```python
from build123d import *

# Parameters (mm, degrees)
SKETCH_1_W                        = 10
SKETCH_1_H                        = 10
EXTRUDE_1_DEPTH                   = 1
SKETCH_2_R                        = 0.5
EXTRUDE_2_DEPTH                   = 5
PATTERN_LINEAR_1_COUNT            = 5
PATTERN_LINEAR_1_PITCH            = 2
PATTERN_LINEAR_2_COUNT            = 5
PATTERN_LINEAR_2_PITCH            = 2
PATTERN_LINEAR_2_COPY_1_SKETCH_R  = 0.5
PATTERN_LINEAR_2_COPY_1_DEPTH     = 5
PATTERN_LINEAR_2_COPY_2_SKETCH_R  = 0.5
PATTERN_LINEAR_2_COPY_2_DEPTH     = 5
PATTERN_LINEAR_2_COPY_3_SKETCH_R  = 0.5
PATTERN_LINEAR_2_COPY_3_DEPTH     = 5
PATTERN_LINEAR_2_COPY_4_SKETCH_R  = 0.5
PATTERN_LINEAR_2_COPY_4_DEPTH     = 5
PATTERN_LINEAR_2_COPY_5_SKETCH_R  = 0.5
PATTERN_LINEAR_2_COPY_5_DEPTH     = 5
PATTERN_LINEAR_2_COPY_6_SKETCH_R  = 0.5
PATTERN_LINEAR_2_COPY_6_DEPTH     = 5
PATTERN_LINEAR_2_COPY_7_SKETCH_R  = 0.5
PATTERN_LINEAR_2_COPY_7_DEPTH     = 5
PATTERN_LINEAR_2_COPY_8_SKETCH_R  = 0.5
PATTERN_LINEAR_2_COPY_8_DEPTH     = 5
PATTERN_LINEAR_2_COPY_9_SKETCH_R  = 0.5
PATTERN_LINEAR_2_COPY_9_DEPTH     = 5
PATTERN_LINEAR_2_COPY_10_SKETCH_R = 0.5
PATTERN_LINEAR_2_COPY_10_DEPTH    = 5
PATTERN_LINEAR_2_COPY_11_SKETCH_R = 0.5
PATTERN_LINEAR_2_COPY_11_DEPTH    = 5
PATTERN_LINEAR_2_COPY_12_SKETCH_R = 0.5
PATTERN_LINEAR_2_COPY_12_DEPTH    = 5
PATTERN_LINEAR_2_COPY_13_SKETCH_R = 0.5
PATTERN_LINEAR_2_COPY_13_DEPTH    = 5
PATTERN_LINEAR_2_COPY_14_SKETCH_R = 0.5
PATTERN_LINEAR_2_COPY_14_DEPTH    = 5
PATTERN_LINEAR_2_COPY_15_SKETCH_R = 0.5
PATTERN_LINEAR_2_COPY_15_DEPTH    = 5
PATTERN_LINEAR_2_COPY_16_SKETCH_R = 0.5
PATTERN_LINEAR_2_COPY_16_DEPTH    = 5


with BuildPart() as part:
    # 草圖1 → 填料-伸長1 (new body)
    with BuildSketch(Plane(origin=(0, 0, 0), x_dir=(1, 0, 0), z_dir=(0, 1, 0))):
        Rectangle(SKETCH_1_W, SKETCH_1_H)
    extrude(amount=EXTRUDE_1_DEPTH)

    # 草圖2 → 填料-伸長2 (add)
    with BuildSketch(Plane(origin=(0, 1, 0), x_dir=(1, 0, 0), z_dir=(0, 1, 0))):
        with Locations(Location((-4, 4, 0), (0, 0, 90))):
            Circle(SKETCH_2_R)
    extrude_2 = extrude(amount=EXTRUDE_2_DEPTH)

    # 直線複製排列1: 填料-伸長2 ×5
    with Locations(*[(i * PATTERN_LINEAR_1_PITCH, 0, 0) for i in range(1, PATTERN_LINEAR_1_COUNT)]):
        add(extrude_2)

    # 直線複製排列2: 填料-伸長2 ×5
    with Locations(*[(0, 0, i * PATTERN_LINEAR_2_PITCH) for i in range(1, PATTERN_LINEAR_2_COUNT)]):
        add(extrude_2)

    # 直線複製排列2 copy 1 sketch → 直線複製排列2 copy 1 (add)
    with BuildSketch(Plane(origin=(2, 1, 2), x_dir=(1, 0, 0), z_dir=(0, 1, 0))):
        with Locations(Location((-4, 4, 0), (0, 0, 90))):
            Circle(PATTERN_LINEAR_2_COPY_1_SKETCH_R)
    extrude(amount=PATTERN_LINEAR_2_COPY_1_DEPTH)

    # 直線複製排列2 copy 2 sketch → 直線複製排列2 copy 2 (add)
    with BuildSketch(Plane(origin=(2, 1, 4), x_dir=(1, 0, 0), z_dir=(0, 1, 0))):
        with Locations(Location((-4, 4, 0), (0, 0, 90))):
            Circle(PATTERN_LINEAR_2_COPY_2_SKETCH_R)
    extrude(amount=PATTERN_LINEAR_2_COPY_2_DEPTH)

    # 直線複製排列2 copy 3 sketch → 直線複製排列2 copy 3 (add)
    with BuildSketch(Plane(origin=(2, 1, 6), x_dir=(1, 0, 0), z_dir=(0, 1, 0))):
        with Locations(Location((-4, 4, 0), (0, 0, 90))):
            Circle(PATTERN_LINEAR_2_COPY_3_SKETCH_R)
    extrude(amount=PATTERN_LINEAR_2_COPY_3_DEPTH)

    # 直線複製排列2 copy 4 sketch → 直線複製排列2 copy 4 (add)
    with BuildSketch(Plane(origin=(2, 1, 8), x_dir=(1, 0, 0), z_dir=(0, 1, 0))):
        with Locations(Location((-4, 4, 0), (0, 0, 90))):
            Circle(PATTERN_LINEAR_2_COPY_4_SKETCH_R)
    extrude(amount=PATTERN_LINEAR_2_COPY_4_DEPTH)

    # 直線複製排列2 copy 5 sketch → 直線複製排列2 copy 5 (add)
    with BuildSketch(Plane(origin=(4, 1, 2), x_dir=(1, 0, 0), z_dir=(0, 1, 0))):
        with Locations(Location((-4, 4, 0), (0, 0, 90))):
            Circle(PATTERN_LINEAR_2_COPY_5_SKETCH_R)
    extrude(amount=PATTERN_LINEAR_2_COPY_5_DEPTH)

    # 直線複製排列2 copy 6 sketch → 直線複製排列2 copy 6 (add)
    with BuildSketch(Plane(origin=(4, 1, 4), x_dir=(1, 0, 0), z_dir=(0, 1, 0))):
        with Locations(Location((-4, 4, 0), (0, 0, 90))):
            Circle(PATTERN_LINEAR_2_COPY_6_SKETCH_R)
    extrude(amount=PATTERN_LINEAR_2_COPY_6_DEPTH)

    # 直線複製排列2 copy 7 sketch → 直線複製排列2 copy 7 (add)
    with BuildSketch(Plane(origin=(4, 1, 6), x_dir=(1, 0, 0), z_dir=(0, 1, 0))):
        with Locations(Location((-4, 4, 0), (0, 0, 90))):
            Circle(PATTERN_LINEAR_2_COPY_7_SKETCH_R)
    extrude(amount=PATTERN_LINEAR_2_COPY_7_DEPTH)

    # 直線複製排列2 copy 8 sketch → 直線複製排列2 copy 8 (add)
    with BuildSketch(Plane(origin=(4, 1, 8), x_dir=(1, 0, 0), z_dir=(0, 1, 0))):
        with Locations(Location((-4, 4, 0), (0, 0, 90))):
            Circle(PATTERN_LINEAR_2_COPY_8_SKETCH_R)
    extrude(amount=PATTERN_LINEAR_2_COPY_8_DEPTH)

    # 直線複製排列2 copy 9 sketch → 直線複製排列2 copy 9 (add)
    with BuildSketch(Plane(origin=(6, 1, 2), x_dir=(1, 0, 0), z_dir=(0, 1, 0))):
        with Locations(Location((-4, 4, 0), (0, 0, 90))):
            Circle(PATTERN_LINEAR_2_COPY_9_SKETCH_R)
    extrude(amount=PATTERN_LINEAR_2_COPY_9_DEPTH)

    # 直線複製排列2 copy 10 sketch → 直線複製排列2 copy 10 (add)
    with BuildSketch(Plane(origin=(6, 1, 4), x_dir=(1, 0, 0), z_dir=(0, 1, 0))):
        with Locations(Location((-4, 4, 0), (0, 0, 90))):
            Circle(PATTERN_LINEAR_2_COPY_10_SKETCH_R)
    extrude(amount=PATTERN_LINEAR_2_COPY_10_DEPTH)

    # 直線複製排列2 copy 11 sketch → 直線複製排列2 copy 11 (add)
    with BuildSketch(Plane(origin=(6, 1, 6), x_dir=(1, 0, 0), z_dir=(0, 1, 0))):
        with Locations(Location((-4, 4, 0), (0, 0, 90))):
            Circle(PATTERN_LINEAR_2_COPY_11_SKETCH_R)
    extrude(amount=PATTERN_LINEAR_2_COPY_11_DEPTH)

    # 直線複製排列2 copy 12 sketch → 直線複製排列2 copy 12 (add)
    with BuildSketch(Plane(origin=(6, 1, 8), x_dir=(1, 0, 0), z_dir=(0, 1, 0))):
        with Locations(Location((-4, 4, 0), (0, 0, 90))):
            Circle(PATTERN_LINEAR_2_COPY_12_SKETCH_R)
    extrude(amount=PATTERN_LINEAR_2_COPY_12_DEPTH)

    # 直線複製排列2 copy 13 sketch → 直線複製排列2 copy 13 (add)
    with BuildSketch(Plane(origin=(8, 1, 2), x_dir=(1, 0, 0), z_dir=(0, 1, 0))):
        with Locations(Location((-4, 4, 0), (0, 0, 90))):
            Circle(PATTERN_LINEAR_2_COPY_13_SKETCH_R)
    extrude(amount=PATTERN_LINEAR_2_COPY_13_DEPTH)

    # 直線複製排列2 copy 14 sketch → 直線複製排列2 copy 14 (add)
    with BuildSketch(Plane(origin=(8, 1, 4), x_dir=(1, 0, 0), z_dir=(0, 1, 0))):
        with Locations(Location((-4, 4, 0), (0, 0, 90))):
            Circle(PATTERN_LINEAR_2_COPY_14_SKETCH_R)
    extrude(amount=PATTERN_LINEAR_2_COPY_14_DEPTH)

    # 直線複製排列2 copy 15 sketch → 直線複製排列2 copy 15 (add)
    with BuildSketch(Plane(origin=(8, 1, 6), x_dir=(1, 0, 0), z_dir=(0, 1, 0))):
        with Locations(Location((-4, 4, 0), (0, 0, 90))):
            Circle(PATTERN_LINEAR_2_COPY_15_SKETCH_R)
    extrude(amount=PATTERN_LINEAR_2_COPY_15_DEPTH)

    # 直線複製排列2 copy 16 sketch → 直線複製排列2 copy 16 (add)
    with BuildSketch(Plane(origin=(8, 1, 8), x_dir=(1, 0, 0), z_dir=(0, 1, 0))):
        with Locations(Location((-4, 4, 0), (0, 0, 90))):
            Circle(PATTERN_LINEAR_2_COPY_16_SKETCH_R)
    extrude(amount=PATTERN_LINEAR_2_COPY_16_DEPTH)


solid = part.part
```
Design review of the part built by this model. Coordinates are the model's own, in mm. A direction names the side the tool comes from. Give positions to 0.01 mm unless a question says otherwise; leave off trailing zeros. Write each loop counter-clockwise with the first axis right and the second up, starting at its lowest first coordinate (ties: lowest second). Pieces come first, ordered by that corner, then holes. Notation, with made-up numbers: (84, 81) -> (110, 81) arc R23 cw to (110, 115) -> close; hole circle Ø4 at (-31, 54). An arc over 180 degrees is marked (long way). Answer in a Markdown table with one row per item.
(1) Consider section C-C (x = -4). State the section outline as (y, z) points, then the cut area to 3 significant figures.
Results:
| item | result |
|---|---|
| outline | (0, -5) -> (1, -5) -> (1, -4.5) -> (6, -4.5) -> (6, -3.5) -> (1, -3.5) -> (1, -2.5) -> (6, -2.5) -> (6, -1.5) -> (1, -1.5) -> (1, -0.5) -> (6, -0.5) -> (6, 0.5) -> (1, 0.5) -> (1, 1.5) -> (6, 1.5) -> (6, 2.5) -> (1, 2.5) -> (1, 3.5) -> (6, 3.5) -> (6, 4.5) -> (1, 4.5) -> (1, 5) -> (0, 5) -> close |
| area | 35.0 mm2 |
(2) Mouldability with a two-part tool opening along Z and no side actions: class faces 1 (the flat face through (2, 6, 2)), 2 (the cylindrical face through (1.7, 3.5, -1.6)) as +Z half, -Z half, draft (parallel to the pull), parting line (faces both ways), or undercut.
Results:
| item | result |
|---|---|
| face 1 | draft |
| face 2 | undercut |
(3) Clearance check with flat-ended pins moving along their axes: pin 1 (1 mm diameter, centred on x = 2.5, y = 5, fed in from +Z); pin 2 (2 mm diameter, centred on y = 5, z = -3, fed in from +X). State where each tip first meets the part, or that it passes through.
Results:
| item | result |
|---|---|
| pin 1 | z = 4.5 |
| pin 2 | x = 4.5 |
(4) Consider section A-A (y = 2.4). Count the separate pieces of the cut face and the enclosed holes in it, then the cut area to 3 significant figures.
Results:
| item | result |
|---|---|
| separate pieces | 25 |
| enclosed holes | 0 |
| area | 19.6 mm2 |
(5) To check wall thickness, follow probe 1 along X at (y, z) = (4.7, -4); probe 2 along X at (y, z) = (4.8, 1.75). State the ranges of each line that lie inside material, in increasing order.
Results:
| item | result |
|---|---|
| probe 1 | -4.5 to -3.5, -2.5 to -1.5, -0.5 to 0.5, 1.5 to 2.5, 3.5 to 4.5 |
| probe 2 | -4.43 to -3.57, -2.43 to -1.57, -0.43 to 0.43, 1.57 to 2.43, 3.57 to 4.43 |
(6) Consider section B-B (z = -4). State the section outline as (x, y) points.
Results:
| item | result |
|---|---|
| outline | (-5, 0) -> (5, 0) -> (5, 1) -> (4.5, 1) -> (4.5, 6) -> (3.5, 6) -> (3.5, 1) -> (2.5, 1) -> (2.5, 6) -> (1.5, 6) -> (1.5, 1) -> (0.5, 1) -> (0.5, 6) -> (-0.5, 6) -> (-0.5, 1) -> (-1.5, 1) -> (-1.5, 6) -> (-2.5, 6) -> (-2.5, 1) -> (-3.5, 1) -> (-3.5, 6) -> (-4.5, 6) -> (-4.5, 1) -> (-5, 1) -> close |
(7) For faces 3 (the flat face through (-4, 6, 4)), 4 (the cylindrical face through (3.504, 3.465, 4.065)), list the 3-axis set-ups (+Z, -Z, +X, -X, +Y, -Y) from which the entire face can be reached by the end or side of a thin tool; tool diameter is ignored.
Results:
| item | result |
|---|---|
| face 3 | +Z, -Z, +X, -X, +Y |
| face 4 | +Y |
(8) Consider section D-D (z = -0.75). State the section outline as (x, y) points, then the cut area to 3 significant figures.
Results:
| item | result |
|---|---|
| outline | (-5, 0) -> (5, 0) -> (5, 1) -> (-5, 1) -> close |
| area | 10.0 mm2 |
